from build123d import *

# Parameters (mm, degrees)
CROQUIS1_R              = 1.075
SALIENTE_EXTRUIR1_DEPTH = 114


with BuildPart() as part:
    # Croquis1 → Saliente-Extruir1 (new body)
    with BuildSketch(Plane.XY):
        Polygon((-1.420025253, 1.915), (-2.8, 3.294974747), (-2.8, 4.1), (-1.625, 4.1), (-2.525, 5), (-5, 5), (-5, 2.52), (-4.1, 1.62), (-4.1, 2.8), (-3.294974747, 2.8), (-1.915, 1.420025253), (-1.915, -1.420025253), (-3.294974747, -2.8), (-4.1, -2.8), (-4.1, -1.625), (-5, -2.525), (-5, -5), (-2.52, -5), (-1.62, -4.1), (-2.8, -4.1), (-2.8, -3.294974747), (-1.420025253, -1.915), (1.420025253, -1.915), (2.8, -3.294974747), (2.8, -4.1), (1.625, -4.1), (2.525, -5), (5, -5), (5, -2.52), (4.1, -1.62), (4.1, -2.8), (3.294974747, -2.8), (1.915, -1.420025253), (1.915, 1.420025253), (3.294974747, 2.8), (4.1, 2.8), (4.1, 1.625), (5, 2.525), (5, 5), (2.52, 5), (1.62, 4.1), (2.8, 4.1), (2.8, 3.294974747), (1.420025253, 1.915), align=None)
        with Locations(Location((0, 0, 0), (0, 0, 180))):
            Circle(CROQUIS1_R, mode=Mode.SUBTRACT)
    extrude(amount=SALIENTE_EXTRUIR1_DEPTH)


solid = part.part
Here's how the part is built. I have some questions about the finished solid (model axes, mm). A direction names the side the tool comes from. Coordinates: 2 decimals unless noted, no trailing zeros. Write each loop counter-clockwise with the first axis right and the second up, starting at its lowest first coordinate (ties: lowest second). Pieces come first, ordered by that corner, then holes.
1) I'm going to push flat-ended pins straight in: pin 1 (3 mm diameter, centred on x = 0.5, z = 75.5, fed in from +Y); pin 2 (2.5 mm diameter, centred on y = -0.5, z = 29.5, fed in from -X) (3 decimals); pin 3 (1.4 mm diameter, centred on x = 0, z = 56.5, fed in from -Y) (3 decimals); pin 4 (1.3 mm diameter, centred on x = 0, y = 0, fed in from -Z). Where does each tip first touch, or does it pass through?
Filled in:
pin 1: stops at y = 4.48
pin 2: stops at x = -4.225
pin 3: stops at y = -1.915
pin 4: passes through
2) Which directions (+Z, -Z, +X, -X, +Y, -Y) give clear straight access to the entire face, cutting with the end or side of a thin tool? Please do faces 4 (the face through (1.915, 0, 56)), 5 (the face through (-1.915, 0, 56)), 6 (the face through (0, -1.915, 56)).
Filled in:
face 4: +Z, -Z, +X
face 5: +Z, -Z, -X
face 6: +Z, -Z, -Y
3) If we section it at A-A (x = 0): List the corners of the cut face in (y, z) for me (3 decimals), plus the area to 3 significant figures.
Filled in:
outline: (-1.915, 0) - (-1.075, 0) - (-1.075, 114) - (-1.915, 114) - close; (1.075, 0) - (1.915, 0) - (1.915, 114) - (1.075, 114) - close
area: 192 mm2
4) If I drill on line 1 (Y direction, x = 0, z = 35) (3 decimals); line 2 (X direction, y = 2.5, z = 39.5) (3 decimals); line 3 (X direction, y = -4, z = 36.5), over which ranges is the centre line in solid material (lowest first)?
Filled in:
line 1: y = -1.915 to -1.075, 1.075 to 1.915
line 2: x = -4.98 to -4.1, -2.995 to -2.005, 2.005 to 2.995, 4.1 to 4.975
line 3: x = -5 to -2.8, 2.8 to 5
5) Thinking about a two-plate mould opening in X: for faces 1 (the face through (-4, 5, 56)), 2 (the face through (5, 4, 56)), 3 (the face through (0, 1.915, 56)), which applies, +X half, -X half, draft (parallel to the pull), parting line (faces both ways), or undercut?
Filled in:
face 1: draft
face 2: +X half
face 3: undercut
